Can you work these out from the model? Positions are in its coordinate system, mm. A direction names the side the tool comes from. Coordinates: 2 decimals unless noted, no trailing zeros. Loops run counter-clockwise (first coordinate to the right, second up) from the corner with the lowest first, then second, coordinate; pieces in that order, holes last.
```python
from build123d import *

# Parameters (mm, degrees)
F0_R      = 2.5
F1_DEPTH  = 2
F2_R      = 3
F5_R      = 3
F10_DEPTH = 1
F13_W     = 20
F13_H     = 5
F14_DEPTH = 25
F15_R     = 4.99999


# Not quite as in the source:
# - a fillet or chamfer is up to 0.001 mm smaller than in the source, because OpenCascade refuses the exact size


with BuildPart() as f1:
    # F0 (on Front) → F1 (new body)
    with BuildSketch(Plane.XZ):
        Circle(F0_R)
    extrude(amount=F1_DEPTH)

    # F4: sweep along a path in F3
    with BuildLine(Plane.XY) as f4_path:
        Line((0, -2), (0, -7))
        ThreePointArc((0, -7), (-1.4644660941, -10.5355339059), (-5, -12))
        Line((-5, -12), (-10, -12))
    # F2 (on face) → F4 (sweep)
    with BuildSketch(Plane.XZ.offset(2)):
        Circle(F2_R)
    sweep(path=f4_path.line)

    # F8: sweep along a path in F7
    with BuildLine(Plane.XZ.offset(12)) as f8_path:
        Line((-10, 0), (-15, 0))
        ThreePointArc((-15, 0), (-22.0710678119, -2.9289321881), (-25, -10))
        Line((-25, -10), (-25, -70))
        ThreePointArc((-25, -70), (-22.0710678119, -77.0710678119), (-15, -80))
        Line((-15, -80), (-0.8816349035, -80))
        ThreePointArc((-0.8816349035, -80), (-0.0133940152, -80.0759612349), (0.8284658131, -80.3015368961))
        Line((0.8284658131, -80.3015368961), (9.3969262079, -83.4202014333))
    # F5 (on face) → F8 (sweep)
    with BuildSketch(Plane(origin=(-10, 0, 0), x_dir=(0, -1, 0), z_dir=(-1, 0, 0))):
        with Locations((12, 0)):
            Circle(F5_R)
    sweep(path=f8_path.line)

    # F9 (on face) → F10 (join)
    with BuildSketch(Plane(origin=(35.1084305953, 0, -12.7784237085), x_dir=(0, 1, 0), z_dir=(0.9396926208, 0, -0.3420201433))):
        with BuildLine():
            Line((-9, -75.1754096629), (-15, -75.1754096629))
            ThreePointArc((-15, -75.1754096629), (-12, -78.1754096629), (-9, -75.1754096629))
        make_face()
    extrude(amount=F10_DEPTH)

    # F12: sweep along a path in F11
    with BuildLine(Plane(origin=(-25.7115043875, 0, -70.6417777248), x_dir=(0.9396926208, 0, -0.3420201433), z_dir=(0.3420201433, 0, 0.9396926208))) as f12_path:
        Line((37.3616114661, -12), (70.1276932376, -34.943057454))
    # F9 (on face) + F8_face (on face) → F12 (sweep)
    with BuildSketch(Plane(origin=(35.1084305953, 0, -12.7784237085), x_dir=(0, 1, 0), z_dir=(0.9396926208, 0, -0.3420201433))):
        with BuildLine():
            Line((-9, -75.1754096629), (-15, -75.1754096629))
            ThreePointArc((-15, -75.1754096629), (-12, -78.1754096629), (-9, -75.1754096629))
        make_face()
    with BuildSketch(Plane(origin=(9.3969262079, -12, -83.4202014333), x_dir=(0, 1, 0), z_dir=(0.9396926208, 0, -0.3420201433))):
        with BuildLine():
            ThreePointArc((3, 0), (0, 3), (-3, 0))
            Line((-3, 0), (3, 0))
        make_face()
    sweep(path=f12_path.line)

    # F13 (on face) → F14 (join)
    with BuildSketch(Plane(origin=(65.8984758481, 0, -23.9850836922), x_dir=(0, 1, 0), z_dir=(0.9396926208, 0, -0.3420201433))):
        with Locations((-34.943057454, -75.1754096629)):
            Rectangle(F13_W, F13_H)
    extrude(amount=F14_DEPTH)

    # F15 (radius 5 in the source; OpenCascade refuses exactly that, so slightly less here)
    f15_edges = [f1.edges().sort_by_distance(p)[0] for p in [
        (52.78818, -44.943057, -96.552882),
        (64.534337, -34.943057, -100.828133),
        (52.78818, -24.943057, -96.552882),
    ]]
    fillet(f15_edges, radius=F15_R)


solid = f1.part
```
Item 1: On a 3-axis mill with a long thin cutter (end or side, diameter ignored), from which of +Z, -Z, +X, -X, +Y, -Y can I reach the whole of each face in a straight line? I mean faces 1 (the face through (-3, -5, 0)), 2 (the face through (-10.1, -9.6, -1.8)), 3 (the face through (52.44, -43.52, -98.03)). Say none if no direction works.
Results are:
face 1: +Y
face 2: none
face 3: +Z, +X, -Y
Item 2: I'm going to push flat-ended pins straight in: P1, Ø4, axis at x = 48, y = -27, coming from the -Z side; P2, Ø6.5, axis at x = 1, z = -1, coming from the +Y side; P3, Ø5, axis at x = -0.5, y = -13.5, coming from the +Z side; P4, Ø4.5, axis at x = 52.5, z = -102.5, coming from the +Y side. Where does each tip first touch, or does it pass through?
Results are:
P1: stops at z = -100.86
P2: stops at y = 0
P3: stops at z = 2.97
P4: stops at y = -24.94
Item 3: Suppose I cut it at A-A, the plane z = -68. Please give me the cut outline in (x, y), plus the area to 3 significant figures.
Results are:
outline: circle Ø6 at (-25, -12)
area: 28.3 mm2
Item 4: I need wall thicknesses on line 1 along Z through (x, y) = (25.5, -22); line 2 along Z through (x, y) = (8, -11.5); line 3 along X through (y, z) = (-9.5, -25.5). Which ranges of each line are inside material? Lowest first, please.
Results are:
line 1: z = -91.13 to -86.41
line 2: z = -86.06 to -79.76
line 3: x = -26.66 to -23.34
Item 5: We'd pull the mould along Z, two halves only. Please class faces 4 (the face through (-23.2, -9.6, -40.4)), 5 (the face through (62.94, -34.8, -102.47)), 6 (the face through (2, -2, 2)): +Z half, -Z half, draft (parallel to the pull), parting line (faces both ways), or undercut.
Results are:
face 4: undercut
face 5: parting line
face 6: draft
Item 6: Suppose I cut it at B-B, the plane y = -5. Please give me the cut outline in (x, z), plus the area to 3 significant figures.
Results are:
outline: circle Ø6 at (0, 0)
area: 28.3 mm2
